The model under review builds one solid part; all positions refer to its coordinate system, in mm. Face numbers are marked on the shaded views. Round coordinates to 2 decimals unless told otherwise and drop trailing zeros. Order: outer loops, then holes, each group sorted by start corner. A loop starts at its lowest first (then second) coordinate and runs counter-clockwise, first axis right, second up. Notation, with made-up numbers: M 59,-38.5 L 94,-38.5 A20 cw 94,-9.5 Z; hole C 76.25,-33 d8. An arc over 180 degrees is marked long. Answer as a JSON object with one key per item and string values. Group by question number.
1) Consider section B-B, the plane x = -2.2. Write out the cut boundary in (y, z).
2) To check wall thickness, follow line 1 (Y direction, x = 0, z = 3.5); line 2 (Z direction, x = 0.05, y = 2.1); line 3 (Y direction, x = -2.3, z = 6). State the ranges of each line that lie inside material, in increasing order.
3) The part is to be moulded in two halves that separate along X. For the marked faces 1 and 2, say which applies: +X half, -X half, draft (parallel to the pull), parting line (faces both ways), or undercut.
4) Consider section A-A, the plane y = 0. Write out the cut boundary in (x, z), then the cut area to 3 significant figures.
5) Consider section D-D, the plane y = -1.65. Write out the cut boundary in (x, z), then the cut area to 3 significant figures.
6) Insertion check: pin 1 Ø0.7 at (x, y) = (0.5, -2) entering from +Z; pin 2 Ø0.7 at (x, y) = (2, 0) entering from -Z. Each pin has a flat end and moves straight along its axis. Give the tip position at first contact, or say it passes through.
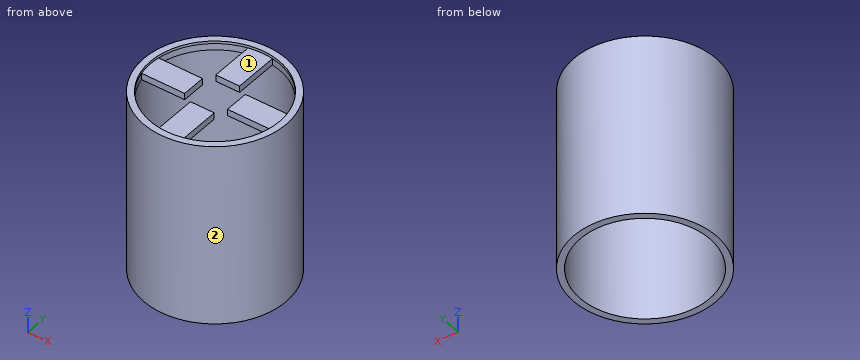
```python
from build123d import *
from build123d.topology import SkipClean

# Parameters (mm, degrees)
ESQUISSE1_R        = 2.749689511
ESQUISSE1_R_2      = 2.5
BOSS_EXTRU_1_DEPTH = 6.7
ESQUISSE2_R        = 2.749689511
BOSS_EXTRU_2_DEPTH = 0.25
ESQUISSE3_R        = 2.749689511
ESQUISSE3_R_2      = 2.5
BOSS_EXTRU_4_DEPTH = 0.1


with BuildPart() as part:
    # Esquisse1 → Boss.-Extru.1 (new body)
    with BuildSketch(Plane.XY):
        Circle(ESQUISSE1_R)
        Circle(ESQUISSE1_R_2, mode=Mode.SUBTRACT)
    extrude(amount=BOSS_EXTRU_1_DEPTH)

    # Esquisse2 → Boss.-Extru.2 (add)
    with SkipClean():  # the faces are left unmerged after this step: merging them gives an invalid solid
        with BuildSketch(Plane.XY.offset(6.7)):
            Circle(ESQUISSE2_R)
            with BuildLine():
                Line((2.439891921, 0.544910465), (0.767744305, 0.544910465))
                Line((0.767744305, 0.544910465), (0.767744305, -0.378691706))
                Line((0.767744305, -0.378691706), (2.471152078, -0.378691706))
                ThreePointArc((2.471152078, -0.378691706), (1.826552736, -1.70695785), (0.544910465, -2.439891921))
                Line((0.544910465, -2.439891921), (0.544910465, -0.767744305))
                Line((0.544910465, -0.767744305), (-0.378691706, -0.767744305))
                Line((-0.378691706, -0.767744305), (-0.378691706, -2.471152078))
                ThreePointArc((-0.378691706, -2.471152078), (-1.70695785, -1.826552736), (-2.439891921, -0.544910465))
                Line((-2.439891921, -0.544910465), (-0.767744305, -0.544910465))
                Line((-0.767744305, -0.544910465), (-0.767744305, 0.378691706))
                Line((-0.767744305, 0.378691706), (-2.471152078, 0.378691706))
                ThreePointArc((-2.471152078, 0.378691706), (-1.826552736, 1.70695785), (-0.544910465, 2.439891921))
                Line((-0.544910465, 2.439891921), (-0.544910465, 0.767744305))
                Line((-0.544910465, 0.767744305), (0.378691706, 0.767744305))
                Line((0.378691706, 0.767744305), (0.378691706, 2.471152078))
                ThreePointArc((0.378691706, 2.471152078), (1.70695785, 1.826552736), (2.439891921, 0.544910465))
            make_face(mode=Mode.SUBTRACT)
        extrude(amount=BOSS_EXTRU_2_DEPTH)

    # Esquisse3 → Boss.-Extru.4 (add)
    with SkipClean():  # the faces are left unmerged after this step: merging them gives an invalid solid
        with BuildSketch(Plane.XY.offset(6.95)):
            Circle(ESQUISSE3_R)
            Circle(ESQUISSE3_R_2, mode=Mode.SUBTRACT)
        extrude(amount=BOSS_EXTRU_4_DEPTH)


solid = part.part
```
Results list:
{
 "1": {"outline": "M -1.65,0 L -1.19,0 L -1.19,7.05 L -1.65,7.05 Z; M -0.54,6.7 L 0.38,6.7 L 0.38,6.95 L -0.54,6.95 Z; M 1.19,0 L 1.65,0 L 1.65,7.05 L 1.19,7.05 Z"},
 "2": {"line 1": "-2.75 to -2.5, 2.5 to 2.75", "line 2": "6.7 to 6.95", "line 3": "-1.51 to -0.98, 0.98 to 1.51"},
 "3": {"face 1": "undercut", "face 2": "parting line"},
 "4": {"outline": "M -2.75,0 L -2.5,0 L -2.5,6.7 L -0.77,6.7 L -0.77,6.95 L -2.5,6.95 L -2.5,7.05 L -2.75,7.05 Z; M 0.77,6.7 L 2.5,6.7 L 2.5,0 L 2.75,0 L 2.75,7.05 L 2.5,7.05 L 2.5,6.95 L 0.77,6.95 Z", "area": "4.39 mm^2"},
 "5": {"outline": "M -2.2,0 L -1.88,0 L -1.88,7.05 L -2.2,7.05 Z; M -0.38,6.7 L 0.54,6.7 L 0.54,6.95 L -0.38,6.95 Z; M 1.88,0 L 2.2,0 L 2.2,7.05 L 1.88,7.05 Z", "area": "4.76 mm^2"},
 "6": {"pin 1": "z = 6.95", "pin 2": "z = 6.7"}
}
